For this review, take the finished solid that the model builds, in its own axes (mm). A direction names the side the tool comes from. Give positions to 0.01 mm unless a question says otherwise; leave off trailing zeros. Loops run counter-clockwise (first coordinate to the right, second up) from the corner with the lowest first, then second, coordinate; pieces in that order, holes last. Notation, with made-up numbers: (85.25, 59.5) - (107.25, 59.5) arc R26 ccw to (107.25, 90.5) - close; hole circle Ø6 at (85.25, 20.25). An arc over 180 degrees is marked (long way). Answer as CSV lines item,"result".
from build123d import *

# Parameters (mm, degrees)
SKETCH1_W           = 46.228
SKETCH1_H           = 62.484
BOSS_EXTRUDE1_DEPTH = 3.175
SKETCH4_W           = 3.175
SKETCH4_H           = 12.954
SKETCH4_H_2         = 5.08
SKETCH4_H_3         = 7.62
SKETCH4_H_4         = 6.35
SKETCH4_W_2         = 8.89
SKETCH4_H_5         = 14.478
CUT_EXTRUDE2_DEPTH  = 4.064
SKETCH5_W           = 39.878
SKETCH5_H           = 4.445
CUT_EXTRUDE3_DEPTH  = 4.064


with BuildPart() as part:
    # Sketch1 → Boss-Extrude1 (new body)
    with BuildSketch(Plane(origin=(0, 0, 0), x_dir=(1, 0, 0), z_dir=(0, 1, 0))):
        with Locations((23.114, 31.242)):
            Rectangle(SKETCH1_W, SKETCH1_H)
    extrude(amount=BOSS_EXTRUDE1_DEPTH)

    # Sketch4 → Cut-Extrude2 (cut)
    with BuildSketch(Plane(origin=(0, 3.175, 0), x_dir=(1, 0, 0), z_dir=(0, 1, 0))):
        with Locations((44.6405, 6.477)):
            Rectangle(SKETCH4_W, SKETCH4_H)
        with Locations((44.6405, 34.544)):
            Rectangle(SKETCH4_W, SKETCH4_H_2)
        with Locations((44.6405, 45.974)):
            Rectangle(SKETCH4_W, SKETCH4_H_2)
        with Locations((44.6405, 58.674)):
            Rectangle(SKETCH4_W, SKETCH4_H_3)
        with Locations((44.6405, 22.479)):
            Rectangle(SKETCH4_W, SKETCH4_H_4)
        with Locations((1.5875, 6.477)):
            Rectangle(SKETCH4_W, SKETCH4_H)
        with Locations((1.5875, 22.479)):
            Rectangle(SKETCH4_W, SKETCH4_H_4)
        with Locations((1.5875, 34.544)):
            Rectangle(SKETCH4_W, SKETCH4_H_2)
        with Locations((1.5875, 45.974)):
            Rectangle(SKETCH4_W, SKETCH4_H_2)
        with Locations((1.5875, 58.674)):
            Rectangle(SKETCH4_W, SKETCH4_H_3)
        with Locations((25.433226228, 22.312235855)):
            Rectangle(SKETCH4_W_2, SKETCH4_H_5)
    extrude(amount=-CUT_EXTRUDE2_DEPTH, mode=Mode.SUBTRACT)

    # Sketch5 → Cut-Extrude3 (cut)
    with BuildSketch(Plane(origin=(0, 3.175, 0), x_dir=(1, 0, 0), z_dir=(0, 1, 0))):
        with Locations((23.114, 60.2615)):
            Rectangle(SKETCH5_W, SKETCH5_H)
    extrude(amount=-CUT_EXTRUDE3_DEPTH, mode=Mode.SUBTRACT)


solid = part.part
1) Draft analysis for pull direction Z (two halves, no side actions). For faces 1 (the flat face through (2, 2, -54.864)), 2 (the flat face through (25, 2, -29.551)), 3 (the flat face through (46.228, 2, -16)), state which applies: pulls with the +Z half, pulls with the -Z half, needs draft (parallel to the pull), parting line crosses it, or undercut.
From the geometry:
face 1,"pulls with the -Z half"
face 2,"undercut"
face 3,"needs draft"
2) Insertion check: P1, Ø1, axis at y = 1.5, z = -46, coming from the -X side (3 decimals); P2, Ø1.6, axis at x = 45, y = 1.5, coming from the +Z side; P3, Ø1.6, axis at y = 2, z = -56.5, coming from the +X side. Each pin has a flat end and moves straight along its axis. Give the tip position at first contact, or say it passes through.
From the geometry:
P1,"stops at x = 3.175"
P2,"stops at z = -12.95"
P3,"stops at x = 43.05"
3) Machinability: for faces 4 (the flat face through (2, 2, -19.304)), 5 (the flat face through (25, 2, -15.073)), 6 (the flat face through (3.175, 2, -6)), which of the approach directions +Z, -Z, +X, -X, +Y, -Y give a long, thin tool a straight path to every point of the face, cutting with its end or side? Answer none if there is none.
From the geometry:
face 4,"-X, +Y, -Y"
face 5,"+Y, -Y"
face 6,"+Z, -X, +Y, -Y"
4) Consider section B-B on z = -46.5. Write out the cut boundary in (x, y) (3 decimals).
From the geometry:
outline,"(3.175, 0) - (43.053, 0) - (43.053, 3.175) - (3.175, 3.175) - close"
5) Consider section A-A on z = -27. Write out the cut boundary in (x, y) (3 decimals), and give its area (3 significant figures).
From the geometry:
outline,"(0, 0) - (20.988, 0) - (20.988, 3.175) - (0, 3.175) - close; (29.878, 0) - (46.228, 0) - (46.228, 3.175) - (29.878, 3.175) - close"
area,"119 mm^2"
6) Wall thickness on line 1 (Z direction, x = 29.5, y = 0.5); line 2 (X direction, y = 1.5, z = -29.5); line 3 (X direction, y = 0.75, z = -46) (3 decimals): over which ranges is each line inside the solid? List them lowest first. Write a range as from..to.
From the geometry:
line 1,"z = -58.04..-29.55, -15.07..0"
line 2,"x = 0..20.99, 29.88..46.23"
line 3,"x = 3.175..43.053"
